from build123d import *

# Parameters (mm, degrees)
F0_R     = 1.35
F0_R_2   = 1.15
F1_DEPTH = 12.73
F3_DEPTH = 25
F4_R     = 5
F5_R     = 3
F6_R     = 3
F7_DEPTH = 1
F8_R     = 3.95
F9_DEPTH = 1


with BuildPart() as f1:
    # F0 (on Top) → F1 (new body)
    with BuildSketch(Plane.XY):
        Polygon((3.75, -4.35), (3.75, 0), (3.75, 27.2), (-8.25, 27.2), (-8.25, 20.45), (-20.25, 20.45), (-20.25, 17.05), (-3.75, 17.05), (-3.75, -1.35), (-20.25, -1.35), (-20.25, -4.35), align=None)
        Circle(F0_R, mode=Mode.SUBTRACT)
        with Locations((-4.6, 23.55)):
            Circle(F0_R_2, mode=Mode.SUBTRACT)
        with Locations((0.1, 23.55)):
            Circle(F0_R_2, mode=Mode.SUBTRACT)
    extrude(amount=F1_DEPTH)

    # F2 (on face) → F3 (cut)
    with BuildSketch(Plane.XZ.offset(4.35)):
        with BuildLine():
            ThreePointArc((-17.35, 6.365), (-15.2, 4.215), (-13.05, 6.365))
            ThreePointArc((-13.05, 6.365), (-15.2, 8.515), (-17.35, 6.365))
        make_face()
    extrude(amount=-F3_DEPTH, mode=Mode.SUBTRACT)

    # F4
    f4_edges = [f1.edges().sort_by_distance(p)[0] for p in [
        (-20.25, -2.85, 12.73),
        (-20.25, 18.75, 12.73),
        (-20.25, -2.85, 0),
        (-20.25, 18.75, 0),
    ]]
    fillet(f4_edges, radius=F4_R)

    # F5
    f5_edges = [f1.edges().sort_by_distance(p)[0] for p in [
        (3.75, -4.35, 6.365),
    ]]
    fillet(f5_edges, radius=F5_R)

    # F6
    f6_edges = [f1.edges().sort_by_distance(p)[0] for p in [
        (-8.25, 27.2, 6.365),
        (3.75, 27.2, 6.365),
    ]]
    fillet(f6_edges, radius=F6_R)

    # F2 (on face) → F7 (join)
    with BuildSketch(Plane.XZ.offset(4.35)):
        with BuildLine():
            ThreePointArc((-11.25, 6.365), (-15.2, 10.315), (-19.15, 6.365))
            ThreePointArc((-19.15, 6.365), (-15.2, 2.415), (-11.25, 6.365))
        make_face()
        with BuildLine():
            ThreePointArc((-17.35, 6.365), (-15.2, 8.515), (-13.05, 6.365))
            ThreePointArc((-13.05, 6.365), (-15.2, 4.215), (-17.35, 6.365))
        make_face(mode=Mode.SUBTRACT)
    extrude(amount=F7_DEPTH)

    # F8 (on face) → F9 (join)
    with BuildSketch(Plane(origin=(0, 20.45, 0), x_dir=(-1, 0, 0), z_dir=(0, 1, 0))):
        with Locations((15.2, 6.365)):
            Circle(F8_R)
        with BuildLine():
            ThreePointArc((13.05, 6.365), (15.2, 8.515), (17.35, 6.365))
            ThreePointArc((17.35, 6.365), (15.2, 4.215), (13.05, 6.365))
        make_face(mode=Mode.SUBTRACT)
    extrude(amount=F9_DEPTH)


solid = f1.part
For this review, take the finished solid that the model builds, in its own axes (mm). A direction names the side the tool comes from. Give positions to 0.01 mm unless a question says otherwise; leave off trailing zeros. Order: outer loops, then holes, each group sorted by start corner. A loop starts at its lowest first (then second) coordinate and runs counter-clockwise, first axis right, second up. Notation, with made-up numbers: M -17,3.25 L 36,3.25 A21 cw 36,10.25 Z; hole C 80,1.5 d1. An arc over 180 degrees is marked long. Answer in a Markdown table with one row per item. Add a question column.
(1) Consider section B-B on x = -9.75. State the section outline as (y, z) points.
(2) Mouldability with a two-part tool opening along Y and no side actions: class faces 1 (the face through (-2, 12, 0)), 2 (the face through (-0.29, -1.32, 6.28)), 3 (the face through (2.89, 26.3, 6.45)) as +Y half, -Y half, draft (parallel to the pull), parting line (faces both ways), or undercut.
(3) For faces 4 (the face through (-12, 17.05, 6)), 5 (the face through (-14.34, 20.94, 2.51)), 6 (the face through (-12.065, -4.843, 8.769)), list the 3-axis set-ups (+Z, -Z, +X, -X, +Y, -Y) from which the entire face can be reached by the end or side of a thin tool; tool diameter is ignored.
(4) For pin 1 (3.5 mm diameter, centred on x = -15.2, z = 6.365, fed in from -Y); pin 2 (3.5 mm diameter, centred on x = 0, y = 0, fed in from +Z); pin 3 (6.5 mm diameter, centred on y = 11, z = 5, fed in from -X); pin 4 (1.5 mm diameter, centred on x = -11, z = 10, fed in from +Y), all flat-tipped, find the tip position at first contact; note any pin that passes through.
(5) Consider section C-C on y = 0. State the section outline as (x, z) points, and give its area (3 significant figures).
(6) Wall thickness on probe 1 along Z at (x, y) = (-15.2, 19.7) (3 decimals); probe 2 along Y at (x, z) = (-17.5, 8); probe 3 along Y at (x, z) = (-4, 10.5): over which ranges is each line inside the solid? List them lowest first. Write a range as [from, to].
(7) Consider section A-A on x = -4.6. State the section outline as (y, z) points.
(8) Consider section D-D on y = 23.55. State the section outline as (x, z) points.
Evaluation:
| question | item | result |
|---|---|---|
| 1 | outline | M -4.35,0 L -1.35,0 L -1.35,12.73 L -4.35,12.73 Z; M 17.05,0 L 20.45,0 L 20.45,12.73 L 17.05,12.73 Z |
| 2 | face 1 | draft |
| 2 | face 2 | undercut |
| 2 | face 3 | +Y half |
| 3 | face 4 | +Z, -Z, -X |
| 3 | face 5 | +Y |
| 3 | face 6 | -Y |
| 4 | pin 1 | passes through |
| 4 | pin 2 | stops at z = 12.73 |
| 4 | pin 3 | stops at x = -3.75 |
| 4 | pin 4 | stops at y = 20.45 |
| 5 | outline | M -3.75,0 L -1.35,0 L -1.35,12.73 L -3.75,12.73 Z; M 1.35,0 L 3.75,0 L 3.75,12.73 L 1.35,12.73 Z |
| 5 | area | 61.1 mm^2 |
| 6 | probe 1 | z = [0, 4.215], [8.515, 12.73] |
| 6 | probe 2 | y = [-5.35, -1.35], [17.05, 21.45] |
| 6 | probe 3 | y = [-4.35, -1.35], [17.05, 22.57], [24.53, 27.2] |
| 7 | outline | M -4.35,0 L -1.35,0 L -1.35,12.73 L -4.35,12.73 Z; M 17.05,0 L 22.4,0 L 22.4,12.73 L 17.05,12.73 Z; M 24.7,0 L 27.2,0 L 27.2,12.73 L 24.7,12.73 Z |
| 8 | outline | M -8.25,0 L -5.75,0 L -5.75,12.73 L -8.25,12.73 Z; M -3.45,0 L -1.05,0 L -1.05,12.73 L -3.45,12.73 Z; M 1.25,0 L 3.75,0 L 3.75,12.73 L 1.25,12.73 Z |
